```python
from build123d import *

# Parameters (mm, degrees)
CROQUIS1_R                  = 4.7625
SALIENTE_EXTRUIR3_DEPTH     = 7
SALIENTE_EXTRUIR4_DEPTH     = 134.48
SALIENTE_EXTRUIR5_OUTLINE_R = 4.7625
SALIENTE_EXTRUIR5_DEPTH     = 7
CORTAR_EXTRUIR1_DEPTH       = 158.75308333
CROQUIS6_R                  = 4.765
CORTAR_EXTRUIR2_DEPTH       = 190
CROQUIS8_R                  = 1.5
CORTAR_EXTRUIR3_DEPTH       = 154


# Read off the part's stored shape, not the designer's step: Saliente-Extruir5
with BuildPart() as part:
    # Croquis1 → Saliente-Extruir3 (new body)
    with BuildSketch(Plane.XY):
        with BuildLine():
            Line((-25.07, -23), (0, -23))
            ThreePointArc((0, -23), (23, 0), (0, 23))
            Line((0, 23), (-25.07, 23))
            Line((-25.07, 23), (-25.07, -23))
        make_face()
        with Locations((0, -15.2375)):
            Circle(CROQUIS1_R, mode=Mode.SUBTRACT)
    extrude(amount=SALIENTE_EXTRUIR3_DEPTH)

    # Croquis3 → Saliente-Extruir4 (add)
    with BuildSketch(Plane.XY.offset(7)):
        with BuildLine():
            Line((0, 23), (-25.07, 23))
            Line((-25.07, 23), (-25.07, 20))
            Line((-25.07, 20), (1.496213225, 20.399741169))
            ThreePointArc((1.496213225, 20.399741169), (19.71970984, -0.502746878), (0, -20))
            Line((0, -20), (-25.07, -20))
            Line((-25.07, -20), (-25.07, -23))
            Line((-25.07, -23), (0, -23))
            ThreePointArc((0, -23), (23, 0), (0, 23))
        make_face()
    extrude(amount=SALIENTE_EXTRUIR4_DEPTH)

    # Saliente-Extruir5 outline → Saliente-Extruir5 (add)
    with BuildSketch(Plane.XY.offset(141.48)):
        with BuildLine():
            Line((-25.07, 23), (-25.07, -23))
            Line((-25.07, -23), (0, -23))
            ThreePointArc((0, -23), (23, 0), (0, 23))
            Line((0, 23), (-25.07, 23))
        make_face()
        with Locations((0, -15.2375)):
            Circle(SALIENTE_EXTRUIR5_OUTLINE_R, mode=Mode.SUBTRACT)
    extrude(amount=SALIENTE_EXTRUIR5_DEPTH)

    # Croquis5 → Cortar-Extruir1 (cut, through all)
    with BuildSketch(Plane.ZY.offset(25.07)):
        with BuildLine():
            Line((31.24, 8), (47.24, 8))
            ThreePointArc((47.24, 8), (55.24, 0), (47.24, -8))
            Line((47.24, -8), (31.24, -8))
            ThreePointArc((31.24, -8), (23.24, 0), (31.24, 8))
        make_face()
        with BuildLine():
            Line((117.24, 8), (101.24, 8))
            ThreePointArc((101.24, 8), (93.24, 0), (101.24, -8))
            Line((101.24, -8), (117.24, -8))
            ThreePointArc((117.24, -8), (125.24, 0), (117.24, 8))
        make_face()
    extrude(amount=-CORTAR_EXTRUIR1_DEPTH, mode=Mode.SUBTRACT)

    # Croquis6 → Cortar-Extruir2 (cut)
    with BuildSketch(Plane.XY.offset(148.48)):
        with Locations((0, 15.2925)):
            Circle(CROQUIS6_R)
    extrude(amount=-CORTAR_EXTRUIR2_DEPTH, mode=Mode.SUBTRACT)

    # Croquis8 → Cortar-Extruir3 (cut)
    with BuildSketch(Plane.XY.offset(148.48)):
        with Locations((-12.07, 9)):
            Circle(CROQUIS8_R)
        with Locations((-12.07, -9)):
            Circle(CROQUIS8_R)
    extrude(amount=-CORTAR_EXTRUIR3_DEPTH, mode=Mode.SUBTRACT)


solid = part.part
```
Source: CAD feature listing. Evaluate the final solid. Frame: model axes, mm. A direction names the side the tool comes from. Give positions to 0.01 mm unless a question says otherwise; leave off trailing zeros. Loops run counter-clockwise (first coordinate to the right, second up) from the corner with the lowest first, then second, coordinate; pieces in that order, holes last. Notation, with made-up numbers: (-15, 24.25) -> (1, 24.25) arc R15 cw to (1, 31.25) -> close; hole circle Ø6 at (49.25, -19.5). An arc over 180 degrees is marked (long way). Use a Markdown table: item, result. Add a question column.
(1) Section query B-B (y = -3). Output: boundary loops of the cut face in (x, z), then the cut area to 3 significant figures.
(2) Section query A-A (z = 109). Output: boundary loops of the cut face in (x, y).
(3) Section query C-C (x = 8). Output: boundary loops of the cut face in (y, z).
(4) Pull-direction query (Y, two-part tool) for faces 1 (the face through (-12, 23, 73)), 2 (the face through (-13, -23, 73)), 3 (the face through (-1.032, -19.887, 3.451)), 4 (the face through (22.994, -0.506, 73.201)); classes: +Y half, -Y half, draft (parallel to the pull), parting line (faces both ways), or undercut.
(5) Section query D-D (z = 127.5). Output: boundary loops of the cut face in (x, y), then the cut area to 3 significant figures.
(6) Ray query, line 1 (Y direction, x = -12, z = 3); line 2 (Z direction, x = -7.5, y = 1); line 3 (Y direction, x = -22, z = 138.5). Return the intervals inside material, ascending.
(7) First-contact query: pin 1 Ø12 at (x, y) = (-13.5, -17.5) entering from -Z; pin 2 Ø1.8 at (x, z) = (20, 111) entering from +Y; pin 3 Ø8.5 at (x, y) = (0, -15.24) entering from -Z; pin 4 Ø3 at (y, z) = (-9.5, 81.5) entering from +X. Flat tips, straight axial feed; report the tip coordinate or a pass-through.
(8) Access query for faces 5 (the face through (20, -8, 109)), 6 (the face through (-3.78, 12.39, 3.55)). Directions: +Z, -Z, +X, -X, +Y, -Y. A direction counts if a zero-diameter tool reaches every point of the face in a straight line with its end or side. Return the directions, or none.
Checked values:
| question | item | result |
|---|---|---|
| 1 | outline | (-25.07, 0) -> (22.8, 0) -> (22.8, 23.82) -> (19.47, 23.82) -> (19.47, 7) -> (-25.07, 7) -> close; (-25.07, 141.48) -> (19.47, 141.48) -> (19.47, 124.66) -> (22.8, 124.66) -> (22.8, 148.48) -> (-25.07, 148.48) -> close; (19.47, 54.66) -> (22.8, 54.66) -> (22.8, 93.82) -> (19.47, 93.82) -> close |
| 1 | area | 913 mm^2 |
| 2 | outline | (-25.07, -23) -> (0, -23) arc R23 ccw to (21.56, -8) -> (17.98, -8) arc R20.25 cw to (0, -20) -> (-25.07, -20) -> close; (-25.07, 20) -> (1.5, 20.4) arc R20.25 cw to (18.19, 8) -> (21.56, 8) arc R23 ccw to (0, 23) -> (-25.07, 23) -> close |
| 3 | outline | (-21.56, 0) -> (21.56, 0) -> (21.56, 148.48) -> (-21.56, 148.48) -> close; hole (-18.13, 7) -> (18.62, 7) -> (18.62, 141.48) -> (-18.13, 141.48) -> close |
| 4 | face 1 | +Y half |
| 4 | face 2 | -Y half |
| 4 | face 3 | undercut |
| 4 | face 4 | parting line |
| 5 | outline | (-25.07, -23) -> (0, -23) arc R23 ccw to (0, 23) -> (-25.07, 23) -> (-25.07, 20) -> (1.5, 20.4) arc R20.25 cw to (0, -20) -> (-25.07, -20) -> close |
| 5 | area | 353 mm^2 |
| 6 | line 1 | -23 to -10.5, -7.5 to 7.5, 10.5 to 23 |
| 6 | line 2 | 0 to 7, 141.48 to 148.48 |
| 6 | line 3 | -23 to -20, 20.05 to 23 |
| 7 | pin 1 | z = 0 |
| 7 | pin 2 | y = 12.81 |
| 7 | pin 3 | through |
| 7 | pin 4 | x = 21.56 |
| 8 | face 5 | +X, -X |
| 8 | face 6 | +Z, -Z |
